```python
from build123d import *

# Parameters (mm, degrees)
BOSS_EXTRUDE1_DEPTH                                  = 3
SKETCH3_R                                            = 2.5
CUT_EXTRUDE1_DEPTH                                   = 3
CSK_FOR_M3_HEX_SOCKET_COUNTERSUNK_CAP_SC_D           = 3.4
CSK_FOR_M3_HEX_SOCKET_COUNTERSUNK_CAP_SC_DEPTH       = 20
CSK_FOR_M3_HEX_SOCKET_COUNTERSUNK_CAP_SC_CSINK_D     = 6.72
CSK_FOR_M3_HEX_SOCKET_COUNTERSUNK_CAP_SC_CSINK_ANGLE = 90
CSK_FOR_M3_HEX_SOCKET_COUNTERSUNK_CAP_SC_TIP         = 1.021463052


with BuildPart() as part:
    # Sketch1 → Boss-Extrude1 (new body)
    with BuildSketch(Plane(origin=(0, 0, 0), x_dir=(1, 0, 0), z_dir=(0, 1, 0))):
        with BuildLine():
            Line((33, -57), (-33, -57))
            ThreePointArc((-33, -57), (-40.071067812, -54.071067812), (-43, -47))
            Line((-43, -47), (-43, 47))
            ThreePointArc((-43, 47), (-40.071067812, 54.071067812), (-33, 57))
            Line((-33, 57), (33, 57))
            ThreePointArc((33, 57), (40.071067812, 54.071067812), (43, 47))
            Line((43, 47), (43, -47))
            ThreePointArc((43, -47), (40.071067812, -54.071067812), (33, -57))
        make_face()
    extrude(amount=BOSS_EXTRUDE1_DEPTH)

    # Sketch3 → Cut-Extrude1 (cut)
    with BuildSketch(Plane.XZ):
        with Locations(Location((0, 31.4, 0), (0, 0, 270))):
            Circle(SKETCH3_R)
    extrude(amount=-CUT_EXTRUDE1_DEPTH, mode=Mode.SUBTRACT)

    # CSK for M3 Hex Socket Countersunk Cap Screw1
    with Locations(Plane(origin=(0, 0, 0), x_dir=(-1, 0, 0), z_dir=(0, -1, 0))):
        with Locations((37, 37), (37, -37), (-37, 37), (-37, -37)):
            CounterSinkHole(CSK_FOR_M3_HEX_SOCKET_COUNTERSUNK_CAP_SC_D / 2, CSK_FOR_M3_HEX_SOCKET_COUNTERSUNK_CAP_SC_CSINK_D / 2, depth=CSK_FOR_M3_HEX_SOCKET_COUNTERSUNK_CAP_SC_DEPTH, counter_sink_angle=CSK_FOR_M3_HEX_SOCKET_COUNTERSUNK_CAP_SC_CSINK_ANGLE)
            with Locations((0, 0, -(CSK_FOR_M3_HEX_SOCKET_COUNTERSUNK_CAP_SC_DEPTH + CSK_FOR_M3_HEX_SOCKET_COUNTERSUNK_CAP_SC_TIP / 2))):  # 118° drill point
                Cone(0, CSK_FOR_M3_HEX_SOCKET_COUNTERSUNK_CAP_SC_D / 2, CSK_FOR_M3_HEX_SOCKET_COUNTERSUNK_CAP_SC_TIP, mode=Mode.SUBTRACT)


solid = part.part
```
Geometry check sheet. Reference: the model listing, model coordinates, mm. Coordinates: 2 decimals unless noted, no trailing zeros. Order: outer loops, then holes, each group sorted by start corner. A loop starts at its lowest first (then second) coordinate and runs counter-clockwise, first axis right, second up. Notation, with made-up numbers: (71.5, -8.5) - (95.5, -8.5) arc R17 cw to (95.5, 22.5) - close; hole circle Ø2 at (-22, 75.25). An arc over 180 degrees is marked (long way). Answer in a Markdown table with one row per item. Add a question column.
1. Section check B-B (x = 0). Enter the section's corners in (y, z), plus the area to 3 significant figures.
2. Gauge pin test, flat ends, axial feed: pin 1 Ø6.5 at (x, z) = (0, 31.4) entering from -Y; pin 2 Ø4.5 at (x, z) = (37, -37) entering from -Y; pin 3 Ø4 at (x, z) = (37, 37) entering from -Y. Record the tip position at first contact, or that the pin passes through.
3. Section check C-C (x = 37). Enter the section's corners in (y, z).
4. Section check A-A (z = -37). Enter the section's corners in (x, y).
5. Draft check along X on faces 1 (the face through (-43, 1, 1)), 2 (the face through (-37.37, 2.34, 38.66)), 3 (the face through (1, 3, -1)), 4 (the face through (43, 1, -1)). Enter one of: +X half, -X half, draft (parallel to the pull), parting line (faces both ways), or undercut.
6. Material ranges on L1, parallel to X at y = 2.65, z = -37; L2, parallel to X at y = 2.2, z = 31.4; L3, parallel to Z at x = 37, y = 2.05, recorded low to high. Write a range as [from, to].
Data:
| question | item | result |
|---|---|---|
| 1 | outline | (0, -57) - (3, -57) - (3, 28.9) - (0, 28.9) - close; (0, 33.9) - (3, 33.9) - (3, 57) - (0, 57) - close |
| 1 | area | 327 mm² |
| 2 | pin 1 | stops at y = 0 |
| 2 | pin 2 | stops at y = 1.11 |
| 2 | pin 3 | stops at y = 1.36 |
| 3 | outline | (0, -56.17) - (3, -56.17) - (3, -38.7) - (1.66, -38.7) - (0, -40.36) - close; (0, -33.64) - (1.66, -35.3) - (3, -35.3) - (3, 35.3) - (1.66, 35.3) - (0, 33.64) - close; (0, 40.36) - (1.66, 38.7) - (3, 38.7) - (3, 56.17) - (0, 56.17) - close |
| 4 | outline | (-43, 0) - (-40.36, 0) - (-38.7, 1.66) - (-38.7, 3) - (-43, 3) - close; (-35.3, 1.66) - (-33.64, 0) - (33.64, 0) - (35.3, 1.66) - (35.3, 3) - (-35.3, 3) - close; (38.7, 1.66) - (40.36, 0) - (43, 0) - (43, 3) - (38.7, 3) - close |
| 5 | face 1 | -X half |
| 5 | face 2 | undercut |
| 5 | face 3 | draft |
| 5 | face 4 | +X half |
| 6 | L1 | x = [-43, -38.7], [-35.3, 35.3], [38.7, 43] |
| 6 | L2 | x = [-43, -2.5], [2.5, 43] |
| 6 | L3 | z = [-56.17, -38.7], [-35.3, 35.3], [38.7, 56.17] |
